Here's how the part is built. I have some questions about the finished solid (model axes, mm). Round coordinates to 2 decimals unless told otherwise and drop trailing zeros. Order: outer loops, then holes, each group sorted by start corner. A loop starts at its lowest first (then second) coordinate and runs counter-clockwise, first axis right, second up. Notation, with made-up numbers: (4.5, 38) -> (32.5, 38) arc R17 ccw to (32.5, 52) -> close; hole circle Ø5 at (68.5, 59.5). An arc over 180 degrees is marked (long way). One line per item, written item: value.
Autodesk Inventor part; units mm, degrees
ref_plane "YZ Plane" through (0, 0, 0) normal (1, 0, 0) x (0, 1, 0)
ref_plane "XZ Plane" through (0, 0, 0) normal (0, 1, 0) x (-1, 0, 0)
ref_plane "XY Plane" through (0, 0, 0) normal (0, 0, 1) x (1, 0, 0)
sketch "Sketch1" plane through (0, 0, 0) normal (0, 1, 0) x (-1, 0, 0)
  line L0 (-16.4, 36.4) -> (17.6, 36.4)
  line L1 (17.6, 2.4) -> (-16.4, 2.4)
  line L2 (0, 36.4) -> (10, 36.4)
  line L3 (16.4, 6.0801) -> (17.6, 6.0801)
  line L4 (10, 24.9) -> (12.1364, 24.9)
  line L5 (-16.4, 2.4) -> (-16.4, 6.0801)
  line L6 (-16.4, 43.7199) -> (-16.4, 36.4)
  line L7 (17.6, 36.4) -> (17.6, 43.7199)
  line L8 (17.6, 6.0801) -> (17.6, 2.4)
  line L9 (0, 36.4) -> (0, 32.7199)
  line L10 (-16.4, 36.4) -> (17.6, 36.4)
  line L11 (17.6, 36.4) -> (17.6, 2.4)
  line L12 (17.6, 2.4) -> (-16.4, 2.4)
  line L13 (-16.4, 2.4) -> (-16.4, 36.4)
  circle A0 centre (-5.2589, 26.3219) radius 2
  line L14 (0, 19.4) -> (0, 2.4)
  circle A1 centre (5.2589, 26.3219) radius 2
  circle A2 centre (-5.2589, 12.4781) radius 2
  circle A3 centre (5.2589, 12.4781) radius 2
  point P0 (0, 0)
  point P1 (10, 2.4)
  point P2 (-10, 47.4)
  point P3 (-10, 2.4)
  point P4 (-17.6, 6.0801)
  point P5 (-17.6, 43.7199)
  point P6 (-10, 24.9)
  dimension "d1" = 34
  dimension "d4" = 10
  dimension "d5" = 4
extrude "Extrusion2" add sketch "Sketch1" along normal blind 9
sketch "Sketch7" plane through (-17.6, 0, 36.4) normal (0, 0, 1) x (1, 0, 0)
  line L0 (0, 0) -> (34, 0)
  line L1 (0, 9) -> (34, 9)
  line L2 (17, 9) -> (17, 0)
  line L3 (0, 9) -> (17, 9)
  circle A0 centre (30.6525, 4.2375) radius 2.0955
  circle A1 centre (7.2, 4.2375) radius 2.0955
  line L4 (18.8525, 9) -> (-33.0985, 9)
  line L5 (18.8525, 23.1318) -> (18.8525, -15.955)
  line L6 (0, 0) -> (0, 9)
  dimension "d16" = 4.7625
  dimension "d21" = 7.2
extrude "Extrusion6" cut sketch "Sketch7" against normal up to next contours A1
sketch "Sketch8" plane through (-17.6, 0, 36.4) normal (0, 0, 1) x (1, 0, 0)
  circle A0 centre (7.2, 4.2375) radius 2.0955
  line L0 (0, 9) -> (34, 9)
  line L1 (0, 0) -> (0, 9)
  line L2 (17, 9) -> (17, 4.5)
  circle A1 centre (7.2, 4.2375) radius 2.0955
  circle A2 centre (26.8, 4.2375) radius 2.0955
  line L3 (34, 0) -> (34, 9)
  point P0 (17.6, 0)
  dimension "d22" = 7.2
  dimension "d23" = 7.2
  dimension "d24" = 19.6
extrude "Extrusion7" cut sketch "Sketch8" against normal up to next contours A2
sketch "Sketch10" plane through (16.4, 0, 2.4) normal (0, 0, -1) x (-1, 0, 0)
  line L0 (0, 0) -> (34, 0)
  line L1 (0, 9) -> (4, 9)
  line L2 (4, 9) -> (4, 0)
  line L3 (4, 0) -> (0, 0)
  line L4 (0, 0) -> (0, 9)
  point P0 (16.4, 0)
  dimension "d25" = 4
extrude "Extrusion8" cut sketch "Sketch10" against normal through all
sketch "Sketch11" plane through (-17.6, 0, 2.4) normal (0, 0, -1) x (-1, 0, 0)
  line L0 (-30, 0) -> (0, 0)
  line L1 (0, 9) -> (-4, 9)
  line L2 (-4, 9) -> (-4, 0)
  line L3 (-4, 0) -> (0, 0)
  line L4 (0, 0) -> (0, 9)
  point P0 (-17.6, 0)
  dimension "d28" = 4
extrude "Extrusion9" cut sketch "Sketch11" against normal through all
sketch "Sketch14" plane through (12.4, 0, 36.4) normal (1, 0, 0) x (0, 0, -1)
  line L0 (0, 0) -> (0, 9)
  line L1 (8.0781, 9) -> (8.0781, 15)
  line L2 (0, 15) -> (8.0781, 15)
  line L3 (0, 0) -> (0, 6.35)
  line L4 (0, 6.35) -> (10.8068, 6.35)
  line L5 (4.039, 15) -> (4.039, 6.35)
  circle A0 centre (4.039, 10.389) radius 4.039
  circle A1 centre (4.039, 10.389) radius 3.175
  point P0 (36.4, 0)
  dimension "d35" = 6.35
  dimension "d36" = 6.35
properties part number "top"
Q1. I want a section at D-D on x = -5.25. Write out the boundary of the cut face in (y, z), then the cut area to 3 significant figures.
Answers:
outline: (0, 2.4) -> (9, 2.4) -> (9, 10.48) -> (0, 10.48) -> close; (0, 14.48) -> (9, 14.48) -> (9, 24.32) -> (0, 24.32) -> close; (0, 28.32) -> (9, 28.32) -> (9, 36.4) -> (0, 36.4) -> close
area: 234 mm2
Q2. I want a section at B-B on x = 9.2. Write out the boundary of the cut face in (y, z), then the cut area to 3 significant figures.
Answers:
outline: (0, 2.4) -> (2.14, 2.4) -> (2.14, 36.4) -> (0, 36.4) -> close; (6.33, 2.4) -> (9, 2.4) -> (9, 36.4) -> (6.33, 36.4) -> close
area: 164 mm2
Q3. I need wall thicknesses on line 1 along Y through (x, z) = (-10.5, 9); line 2 along X through (y, z) = (3.25, 13); line 3 along Z through (x, y) = (-6, 4.25). Which ranges of each line are inside material? Lowest first, please.
Answers:
line 1: 0 to 2.14, 6.33 to 9
line 2: -13.6 to -12.25, -8.55 to -7.19, -3.33 to 3.33, 7.19 to 7.35, 11.05 to 12.4
line 3: 2.4 to 10.62, 14.34 to 24.46, 28.18 to 36.4
Q4. I want a section at A-A on z = 11. Write out the boundary of the cut face in (x, y), then the cut area to 3 significant figures.
Answers:
outline: (-13.6, 0) -> (-6.61, 0) -> (-6.61, 9) -> (-13.6, 9) -> close; (-3.91, 0) -> (3.91, 0) -> (3.91, 9) -> (-3.91, 9) -> close; (6.61, 0) -> (12.4, 0) -> (12.4, 9) -> (6.61, 9) -> close; hole circle Ø4.19 at (-10.4, 4.24); hole circle Ø4.19 at (9.2, 4.24)
area: 158 mm2
Q5. I want a section at C-C on y = 3.25. Write out the boundary of the cut face in (x, z), then the cut area to 3 significant figures.
Answers:
outline: (-13.6, 2.4) -> (-12.25, 2.4) -> (-12.25, 36.4) -> (-13.6, 36.4) -> close; (-8.55, 2.4) -> (7.35, 2.4) -> (7.35, 36.4) -> (-8.55, 36.4) -> close; (11.05, 2.4) -> (12.4, 2.4) -> (12.4, 36.4) -> (11.05, 36.4) -> close; hole circle Ø4 at (-5.26, 12.48); hole circle Ø4 at (-5.26, 26.32); hole circle Ø4 at (5.26, 12.48); hole circle Ø4 at (5.26, 26.32)
area: 582 mm2
Q6. If we mould it in two halves opening along Z, with no side actions, what happens to faces 1 (the face through (12.4, 5, 19)), 2 (the face through (0, 4, 36.4)), 3 (the face through (-6.182, 4.437, 14.252))? For each: pulls with the +Z half, pulls with the -Z half, needs draft (parallel to the pull), parting line crosses it, or undercut.
Answers:
face 1: needs draft
face 2: pulls with the +Z half
face 3: undercut
Q7. For P1, Ø12, axis at x = -4, z = 16.5, coming from the -Y side; P2, Ø3, axis at x = 5.26, z = 12.48, coming from the -Y side, each with a flat end and sliding along its axis, tell me the tip position at first contact or that it passes through.
Answers:
P1: y = 0
P2: through
